Input: part model. Units: mm. Frame: model coordinates. A direction names the side the tool comes from. Round coordinates to 2 decimals unless told otherwise and drop trailing zeros. Loops run counter-clockwise (first coordinate to the right, second up) from the corner with the lowest first, then second, coordinate; pieces in that order, holes last. Notation, with made-up numbers: M 76.5,71 L 98.5,71 A33 ccw 98.5,102 Z; hole C 89,32 d5. An arc over 180 degrees is marked long. Put each result on its own line as item: value. Start each with the question number.
1) Section B-B on z = 23. Output: boundary loops of the cut face in (x, y).
2) Section C-C on x = 7.5. State how many separate pieces and enclosed holes the cut face has, plus the area to 3 significant figures.
3) Pin query (flat end, axial travel): pin 1 (4 mm diameter, centred on x = 6, z = 26, fed in from -Y); pin 2 (3 mm diameter, centred on x = 7, y = -13.5, fed in from +Z); pin 3 (4.5 mm diameter, centred on x = 7, z = 32.5, fed in from +Y). Return the tip coordinate at first contact, or that it passes through.
4) Reachability of faces 4 (the face through (7, 13, 6)), 5 (the face through (5, 0.6, 34)), 6 (the face through (7, -10, 22)), 7 (the face through (9, 5.6, 31)) from +Z, -Z, +X, -X, +Y, -Y: full face, straight path, thin tool, end or side. Return the list, or none.
5) Section A-A on y = -16. Output: boundary loops of the cut face in (x, z), plus the area to 3 significant figures.
6) Line query: probe 1 along Y at (x, z) = (7, 4.7); probe 2 along Y at (x, z) = (12.25, 31); probe 3 along X at (y, z) = (2.1, 32.5). Output: solid intervals per line, ascending.
7) Section D-D on z = 32.5. Output: boundary loops of the cut face in (x, y), plus the area to 3 significant figures.
8) Draft query along Y for faces 1 (the face through (0, 0, 14)), 2 (the face through (9.62, -15.17, 2.96)), 3 (the face through (7, -21, 3)). Return one class per face: +Y half, -Y half, draft (parallel to the pull), parting line (faces both ways), or undercut.
from build123d import *

# Parameters (mm, degrees)
OBJ1_R           = 2.75
OBJ1_DEPTH       = 8
OBJ2           = 2.75
OBJ3       = 8
TBOLT_SHAFT_R          = 2
TBOLT_SHAFT_DEPTH      = 22
TBOLT_SHAFT_ROLL_ANGLE = 90
UP_SEP_W               = 16
UP_SEP_H               = 1.2
UP_SEP_DEPTH           = 15.5
SHAFT_HOLE_R           = 6
SHAFT_HOLE_DEPTH       = 16
SHAFT_HOLE_PITCH_ANGLE = 90
TBOLT_HEAD_R           = 3.85
TBOLT_HEAD_DEPTH       = 5.4
TBOLT_HEAD_ROLL_ANGLE  = 90
SIDE_BOX_L_W           = 14
SIDE_BOX_L_H           = 11
SIDE_BOX_L_DEPTH       = 31.5
SIDE_BOX_R_W           = 14
SIDE_BOX_R_H           = 11
SIDE_BOX_R_DEPTH       = 31.5
TOTAL_BOX_W            = 14
TOTAL_BOX_H            = 42
TOTAL_BOX_DEPTH        = 37.5


with BuildPart() as obj1:
    # obj1 → obj1 (new body)
    with BuildSketch(Plane(origin=(7, -16, -1), x_dir=(1, 0, 0), z_dir=(0, 0, 1))):
        Circle(OBJ1_R)
    extrude(amount=OBJ1_DEPTH)


with BuildPart() as obj4:
    with BuildSketch(Plane(origin=(7, 16, -1), x_dir=(1, 0, 0), z_dir=(0, 0, 1))):
        Circle(OBJ2)
    extrude(amount=OBJ3)

    # obj4: union obj1
    add(obj1.part)


with BuildPart() as tbolt_shaft:
    # tbolt_shaft → tbolt_shaft (new body)
    with BuildSketch(Plane.XY):
        Circle(TBOLT_SHAFT_R)
    extrude(amount=TBOLT_SHAFT_DEPTH)


with BuildPart() as tbolt_shaft_1:
    # tbolt_shaft roll: moved
    add(tbolt_shaft.part.rotate(Axis((0, 0, 0), (1, 0, 0)), TBOLT_SHAFT_ROLL_ANGLE))


with BuildPart() as tbolt_shaft_2:
    # tbolt_shaft placement: moved
    add(tbolt_shaft_1.part.moved(Location((7, 11, 32.5))))


with BuildPart() as up_sep:
    # up_sep → up_sep (new body)
    with BuildSketch(Plane(origin=(-1, -0.6, 24), x_dir=(1, 0, 0), z_dir=(0, 0, 1))):
        with Locations((8, 0.6)):
            Rectangle(UP_SEP_W, UP_SEP_H)
    extrude(amount=UP_SEP_DEPTH)


with BuildPart() as shaft_hole:
    # shaft_hole → shaft_hole (new body)
    with BuildSketch(Plane.XY):
        Circle(SHAFT_HOLE_R)
    extrude(amount=SHAFT_HOLE_DEPTH)


with BuildPart() as shaft_hole_1:
    # shaft_hole pitch: moved
    add(shaft_hole.part.rotate(Axis((0, 0, 0), (0, 1, 0)), SHAFT_HOLE_PITCH_ANGLE))


with BuildPart() as shaft_hole_2:
    # shaft_hole placement: moved
    add(shaft_hole_1.part.moved(Location((-1, 0, 23))))


with BuildPart() as fuse_shaft_holes:
    # tbolt_head → tbolt_head (new body)
    with BuildSketch(Plane.XY):
        Circle(TBOLT_HEAD_R)
    extrude(amount=TBOLT_HEAD_DEPTH)


with BuildPart() as fuse_shaft_holes_1:
    # tbolt_head roll: moved
    add(fuse_shaft_holes.part.rotate(Axis((0, 0, 0), (1, 0, 0)), TBOLT_HEAD_ROLL_ANGLE))


with BuildPart() as fuse_shaft_holes_2:
    # tbolt_head placement: moved
    add(fuse_shaft_holes_1.part.moved(Location((7, 11, 32.5))))

    # fuse_shaft_holes: union tbolt_shaft, up_sep, shaft_hole
    add(tbolt_shaft_2.part)
    add(up_sep.part)
    add(shaft_hole_2.part)


with BuildPart() as side_box_l:
    # side_box_l → side_box_l (new body)
    with BuildSketch(Plane(origin=(0, -21, 6), x_dir=(1, 0, 0), z_dir=(0, 0, 1))):
        with Locations((7, 5.5)):
            Rectangle(SIDE_BOX_L_W, SIDE_BOX_L_H)
    extrude(amount=SIDE_BOX_L_DEPTH)


with BuildPart() as side_boxes:
    # side_box_r → side_box_r (new body)
    with BuildSketch(Plane(origin=(0, 10, 6), x_dir=(1, 0, 0), z_dir=(0, 0, 1))):
        with Locations((7, 5.5)):
            Rectangle(SIDE_BOX_R_W, SIDE_BOX_R_H)
    extrude(amount=SIDE_BOX_R_DEPTH)

    # side_boxes: union side_box_l
    add(side_box_l.part)


with BuildPart() as sk_final:
    # total_box → total_box (new body)
    with BuildSketch(Plane(origin=(0, -21, 0), x_dir=(1, 0, 0), z_dir=(0, 0, 1))):
        with Locations((7, 21)):
            Rectangle(TOTAL_BOX_W, TOTAL_BOX_H)
    extrude(amount=TOTAL_BOX_DEPTH)

    # sk_shape: cut side_boxes
    add(side_boxes.part, mode=Mode.SUBTRACT)

    # sk_shape_w_holes: cut fuse_shaft_holes
    add(fuse_shaft_holes_2.part, mode=Mode.SUBTRACT)

    # sk_final: cut obj4
    add(obj4.part, mode=Mode.SUBTRACT)


solid = sk_final.part
Geometry results:
1. outline: M 0,-10 L 14,-10 L 14,-6 L 0,-6 Z; M 0,6 L 14,6 L 14,10 L 0,10 Z
2. separate pieces: 5
2. enclosed holes: 0
2. area: 604 mm²
3. pin 1: stops at y = -10
3. pin 2: stops at z = 6
3. pin 3: stops at y = 5.6
4. face 4: +Z, +X, -X, +Y
4. face 5: +Z, +X, -X
4. face 6: +Z, +X, -X, -Y
4. face 7: +Y
5. outline: M 0,0 L 4.25,0 L 4.25,6 L 0,6 Z; M 9.75,0 L 14,0 L 14,6 L 9.75,6 Z
5. area: 51.0 mm²
6. probe 1: y = -21 to -18.75, -13.25 to 13.25, 18.75 to 21
6. probe 2: y = -10 to -0.6, 0.6 to 10
6. probe 3: x = 0 to 5, 9 to 14
7. outline: M 0,-10 L 5,-10 L 5,-0.6 L 0,-0.6 Z; M 0,0.6 L 5,0.6 L 5,5.6 L 3.15,5.6 L 3.15,10 L 0,10 Z; M 9,-10 L 14,-10 L 14,-0.6 L 9,-0.6 Z; M 9,0.6 L 14,0.6 L 14,10 L 10.85,10 L 10.85,5.6 L 9,5.6 Z
7. area: 172 mm²
8. face 1: draft
8. face 2: undercut
8. face 3: -Y half
